```python
from build123d import *

# Parameters (mm, degrees)
F0_R     = 25
F0_R_2   = 15
F1_DEPTH = 80
F3_DEPTH = 80.001
F5_DEPTH = 5
F6_W     = 105.9157028794
F6_H     = 79.6656981111
F7_DEPTH = 60
F8_R     = 17
F9_DEPTH = 20.001


with BuildPart() as f1:
    # F0 (on Top) → F1 (new body)
    with BuildSketch(Plane.XY):
        Circle(F0_R)
        Circle(F0_R_2, mode=Mode.SUBTRACT)
    extrude(amount=F1_DEPTH)

    # F2 (on face) → F3 (cut, through all)
    with BuildSketch(Plane.XY.offset(80)):
        with BuildLine():
            Line((0, 25), (0, 20))
            ThreePointArc((0, 20), (8.7875598508, 17.9660455267), (15.7877700348, 12.2778791869))
            Line((15.7877700348, 12.2778791869), (19.7347125435, 15.3473489836))
            ThreePointArc((19.7347125435, 15.3473489836), (10.9844498135, 22.4575569084), (0, 25))
        make_face()
        with BuildLine():
            Line((-6.1376971007, 19.0349329996), (-7.6721213759, 23.7936662495))
            ThreePointArc((-7.6721213759, 23.7936662495), (-17.3462974082, 18.0029432657), (-23.4923155196, 8.5505035831))
            Line((-23.4923155196, 8.5505035831), (-18.7938524157, 6.8404028665))
            ThreePointArc((-18.7938524157, 6.8404028665), (-13.8770379265, 14.4023546125), (-6.1376971007, 19.0349329996))
        make_face()
        with BuildLine():
            Line((-19.9995793719, -0.1297110174), (-24.9994742148, -0.1621387717))
            ThreePointArc((-24.9994742148, -0.1621387717), (-22.3858443864, -11.1298684228), (-15.2190357252, -19.8338335073))
            Line((-15.2190357252, -19.8338335073), (-12.1752285802, -15.8670668058))
            ThreePointArc((-12.1752285802, -15.8670668058), (-17.9086755091, -8.9038947382), (-19.9995793719, -0.1297110174))
        make_face()
        with BuildLine():
            ThreePointArc((-7.362852386, -23.8911783875), (3.8831909406, -24.6965752306), (14.3394109088, -20.4788011072))
            Line((14.3394109088, -20.4788011072), (11.471528727, -16.3830408858))
            ThreePointArc((11.471528727, -16.3830408858), (3.1065527525, -19.7572601845), (-5.8902819088, -19.11294271))
            Line((-5.8902819088, -19.11294271), (-7.362852386, -23.8911783875))
        make_face()
        with BuildLine():
            ThreePointArc((25, 0), (24.7090377617, 3.8030846547), (23.8429237687, 7.5176449876))
            Line((23.8429237687, 7.5176449876), (19.074339015, 6.0141159901))
            ThreePointArc((19.074339015, 6.0141159901), (19.7769923674, -2.9783507013), (16.4570955105, -11.3650344196))
            Line((16.4570955105, -11.3650344196), (20.5713693881, -14.2062930245))
            ThreePointArc((20.5713693881, -14.2062930245), (23.8671765685, -7.4402878068), (25, 0))
        make_face()
    extrude(amount=-F3_DEPTH, mode=Mode.SUBTRACT)

    # F4 (on face) → F5 (join)
    with BuildSketch(Plane.XY.offset(80)):
        with BuildLine():
            ThreePointArc((19.7347125435, 15.3473489836), (22.1377203615, 11.6155644372), (23.8429237687, 7.5176449876))
            Line((23.8429237687, 7.5176449876), (28.6115085224, 9.0211739851))
            ThreePointArc((28.6115085224, 9.0211739851), (26.5652644339, 13.9386773246), (23.6816550522, 18.4168187804))
            Line((23.6816550522, 18.4168187804), (19.7347125435, 15.3473489836))
        make_face()
        with BuildLine():
            ThreePointArc((-7.6721213759, 23.7936662495), (-3.8831909406, 24.6965752306), (0, 25))
            Line((0, 25), (0, 30))
            ThreePointArc((0, 30), (-4.6598291287, 29.6358902767), (-9.2065456511, 28.5523994994))
            Line((-9.2065456511, 28.5523994994), (-7.6721213759, 23.7936662495))
        make_face()
        with BuildLine():
            ThreePointArc((-25, 0), (-24.6201938253, 4.3412044417), (-23.4923155196, 8.5505035831))
            Line((-23.4923155196, 8.5505035831), (-28.1907786236, 10.2606042998))
            ThreePointArc((-28.1907786236, 10.2606042998), (-29.5442325904, 5.20944533), (-30, 0))
            Line((-30, 0), (-25, 0))
        make_face()
        with BuildLine():
            Line((-8.8354228632, -28.669414065), (-7.362852386, -23.8911783875))
            ThreePointArc((-7.362852386, -23.8911783875), (-11.471744834, -22.2125881082), (-15.2190357252, -19.8338335073))
            Line((-15.2190357252, -19.8338335073), (-18.2628428703, -23.8006002087))
            ThreePointArc((-18.2628428703, -23.8006002087), (-13.7660938008, -26.6551057298), (-8.8354228632, -28.669414065))
        make_face()
        with BuildLine():
            Line((24.6856432657, -17.0475516294), (20.5713693881, -14.2062930245))
            ThreePointArc((20.5713693881, -14.2062930245), (17.7349015968, -17.620251569), (14.3394109088, -20.4788011072))
            Line((14.3394109088, -20.4788011072), (17.2072930905, -24.5745613287))
            ThreePointArc((17.2072930905, -24.5745613287), (21.2818819161, -21.1443018827), (24.6856432657, -17.0475516294))
        make_face()
        with BuildLine():
            Line((-4.6032728256, 14.2761997497), (-6.1376971007, 19.0349329996))
            ThreePointArc((-6.1376971007, 19.0349329996), (-13.8770379265, 14.4023546125), (-18.7938524157, 6.8404028665))
            Line((-18.7938524157, 6.8404028665), (-14.0953893118, 5.1303021499))
            ThreePointArc((-14.0953893118, 5.1303021499), (-10.4077784449, 10.8017659594), (-4.6032728256, 14.2761997497))
        make_face()
        with BuildLine():
            Line((11.8408275261, 9.2084093902), (15.7877700348, 12.2778791869))
            ThreePointArc((15.7877700348, 12.2778791869), (8.7875598508, 17.9660455267), (0, 20))
            Line((0, 20), (0, 15))
            ThreePointArc((0, 15), (6.5906698881, 13.4745341451), (11.8408275261, 9.2084093902))
        make_face()
        with BuildLine():
            ThreePointArc((16.4570955105, -11.3650344196), (19.7769923674, -2.9783507013), (19.074339015, 6.0141159901))
            Line((19.074339015, 6.0141159901), (14.3057542612, 4.5105869926))
            ThreePointArc((14.3057542612, 4.5105869926), (14.825422657, 2.2818507928), (15, 0))
            ThreePointArc((15, 0), (14.3203059411, -4.4641726841), (12.3428216329, -8.5237758147))
            Line((12.3428216329, -8.5237758147), (16.4570955105, -11.3650344196))
        make_face()
        with BuildLine():
            ThreePointArc((-5.8902819088, -19.11294271), (3.1065527525, -19.7572601845), (11.471528727, -16.3830408858))
            Line((11.471528727, -16.3830408858), (8.6036465453, -12.2872806643))
            ThreePointArc((8.6036465453, -12.2872806643), (2.3299145644, -14.8179451383), (-4.4177114316, -14.3347070325))
            Line((-4.4177114316, -14.3347070325), (-5.8902819088, -19.11294271))
        make_face()
    extrude(amount=-F5_DEPTH)

    # F6 (on Top) → F7 (cut)
    with BuildSketch(Plane.XY):
        with Locations((1.6787797213, 0.4578493536)):
            Rectangle(F6_W, F6_H)
    extrude(amount=F7_DEPTH, mode=Mode.SUBTRACT)

    # F8 (on face) → F9 (cut, through all)
    with BuildSketch(Plane.XY.offset(80)):
        Circle(F8_R)
    extrude(amount=-F9_DEPTH, mode=Mode.SUBTRACT)


solid = f1.part
```
Part model, mm, in its own coordinate system. A direction names the side the tool comes from. Coordinates: 2 decimals unless noted, no trailing zeros. Order: outer loops, then holes, each group sorted by start corner. A loop starts at its lowest first (then second) coordinate and runs counter-clockwise, first axis right, second up. Notation, with made-up numbers: (55.5, -7) - (65.5, -7) arc R32 ccw to (65.5, 28) - close; hole circle Ø4 at (31.25, 71). An arc over 180 degrees is marked (long way). Return JSON: item names as keys, results as strings. Group by question number.
Item 1: Which spindle directions (+Z, -Z, +X, -X, +Y, -Y) get a long thin tool onto all of the face, cutting with end or side? Do faces 1 (the face through (-13, -24, 75)), 2 (the face through (-13.97, 14.31, 70.14)), 3 (the face through (17.691, -17.664, 67.395)). Say none if no direction does.
Item 2: Drill centre lines: probe 1 along Y at (x, z) = (-0.5, 73) (3 decimals); probe 2 along X at (y, z) = (0.5, 67.5) (3 decimals); probe 3 along Y at (x, z) = (-3, 61.25). Where is each one in solid material? Low to high. Write a range as from..to.
Item 3: Cut at C-C (x = 25.5). List the corners of the cut face in (y, z).
Item 4: Cut at B-B (x = 13). List the corners of the cut face in (y, z), plus the area to 3 significant figures.
Item 5: Pull direction Y, two halves, no side cores. Call faces 4 (the face through (19, -19, 75)), 5 (the face through (22.716, 7.162, 72.362)), 6 (the face through (-4.595, 29.646, 77.535)): pulls with the +Y half, pulls with the -Y half, needs draft (parallel to the pull), parting line crosses it, or undercut.
Item 6: Cut at A-A (z = 63.25). List the corners of the cut face in (x, y), plus the area to 3 significant figures.
Item 7: Pin check, flat tips, straight feed: pin 1 (1 mm diameter, centred on x = 1, y = 20, fed in from -Z); pin 2 (4 mm diameter, centred on x = 3, z = 62.5, fed in from -Y) (3 decimals); pin 3 (4 mm diameter, centred on x = -26.5, z = 76.5, fed in from -Y); pin 4 (1 mm diameter, centred on x = 12, z = 76.5, fed in from +Y). Stop position of each tip, or through.
Check values:
{
 "1": {"face 1": "-Z, -X, -Y", "face 2": "+Z, -Z", "face 3": "-Z, +X, -Y"},
 "2": {"probe 1": "y = -19.994..-16.993, 16.993..24.995", "probe 2": "x = -24.995..-16.993, 16.993..19.994", "probe 3": "y = -19.77..-16.73, 16.73..24.82"},
 "3": {"outline": "(8.04, 75) - (15.8, 75) - (15.8, 80) - (8.04, 80) - close"},
 "4": {"outline": "(-18.57, 60) - (-10.95, 60) - (-10.95, 80) - (-18.57, 80) - close; (10.95, 60) - (15.2, 60) - (15.2, 80) - (10.95, 80) - close", "area": "237 mm2"},
 "5": {"face 4": "needs draft", "face 5": "undercut", "face 6": "pulls with the +Y half"},
 "6": {"outline": "(-25, -0.16) - (-20, -0.13) arc R20 ccw to (-12.18, -15.87) - (-15.22, -19.83) arc R25 ccw to (-7.36, -23.89) - (-5.89, -19.11) arc R20 ccw to (11.47, -16.38) - (14.34, -20.48) arc R25 ccw to (20.57, -14.21) - (16.46, -11.37) arc R20 ccw to (19.07, 6.01) - (23.84, 7.52) arc R25 ccw to (19.73, 15.35) - (15.79, 12.28) arc R20 ccw to (0, 20) - (0, 25) arc R25 ccw to (-7.67, 23.79) - (-6.14, 19.03) arc R20 ccw to (-18.79, 6.84) - (-23.49, 8.55) arc R25 ccw to start; hole circle Ø34 at (0, 0)", "area": "544 mm2"},
 "7": {"pin 1": "stops at z = 60", "pin 2": "stops at y = -19.975", "pin 3": "stops at y = -0.16", "pin 4": "stops at y = 16.36"}
}
